Can you work these out from the model? Positions are in its coordinate system, mm. Face numbers are marked on the shaded views. A direction names the side the tool comes from. Coordinates: 2 decimals unless noted, no trailing zeros. Order: outer loops, then holes, each group sorted by start corner. A loop starts at its lowest first (then second) coordinate and runs counter-clockwise, first axis right, second up. Notation, with made-up numbers: (-5, 54.5) -> (13, 54.5) arc R28 ccw to (13, 79.5) -> close; hole circle Ø10 at (46.5, -27.75). An arc over 180 degrees is marked (long way). Return JSON: item names as keys, results as strings. Group by question number.
1) If we section it at A-A, the plane z = -2.5: Please give me the cut outline in (x, y), then the cut area to 3 significant figures.
2) For the marked faces 1 and 2, which set-ups out of +Z, -Z, +X, -X, +Y, -Y let a thin tool reach every point of the face, with its end or its side?
3) For pin 1 (5 mm diameter, centred on x = -14, z = -14, fed in from +Y); pin 2 (4 mm diameter, centred on y = 15.5, z = -8, fed in from -X); pin 3 (10 mm diameter, centred on y = -16, z = -16, fed in from -X); pin 4 (12 mm diameter, centred on x = -0.5, y = 21, fed in from -Z), each with a flat end and sliding along its axis, tell me the tip position at first contact or that it passes through.
4) If I drill on probe 1 along Z at (x, y) = (5.5, -5); probe 2 along Z at (x, y) = (24.5, -13); probe 3 along Y at (x, z) = (25, -3), over which ranges is the centre line in solid material (lowest first)? Write a range as from..to.
5) Thinking about a two-plate mould opening in Y: for the marked faces 3, 4 and 5, which applies, +Y half, -Y half, draft (parallel to the pull), parting line (faces both ways), or undercut?
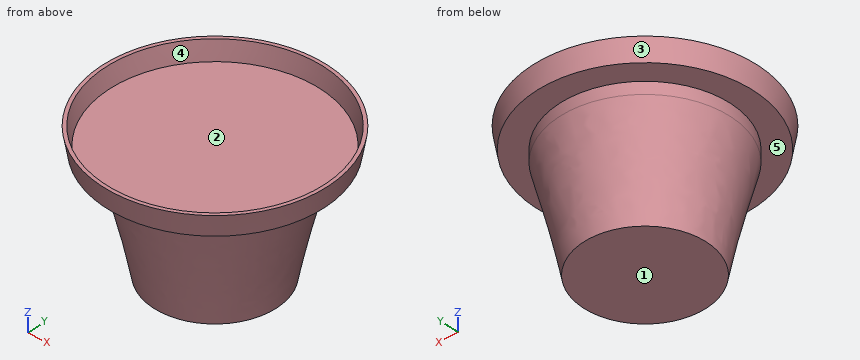
from build123d import *

# Parameters (mm, degrees)
IZIM3_R                     = 25.05
Y_KSEKLIK_EKSTR_ZYON1_DEPTH = 3.5


with BuildPart() as part:
    # Çizim2 → Döndür1 (revolve)
    with BuildSketch(Plane(origin=(0, 0, 0), x_dir=(1, 0, 0), z_dir=(0, 1, 0)), mode=Mode.PRIVATE) as d_nd_r1_sk:
        Polygon((-33, 0), (-31.889140022, 6.3), (-30.889140022, 6.3), (0, 6.3), (0, 5.3), (-30.889140022, 5.3), (-32, 0), align=None)
    revolve(d_nd_r1_sk.sketch.rotate(Axis((0, 0, 0), (0, 0, -1)), 180), axis=Axis((0, 0, 0), (0, 0, -1)))

    # Çizim3 → Yükseklik-Ekstrüzyon1 (add)
    with BuildSketch(Plane(origin=(0, 0, -6.3), x_dir=(-1, 0, 0), z_dir=(0, 0, -1))):
        Circle(IZIM3_R)
    extrude(amount=Y_KSEKLIK_EKSTR_ZYON1_DEPTH)

    # Loft1: read off the stored shape, not the designer's step
    # Loft1: loft between two sections, ruled curve by curve
    loft1_from = [
        Edge.make_bspline([(11.664244151, 13.709318305, -39.8), (-15.754392459, 37.037806607, -39.8), (-39.082880761, 9.619169997, -39.8), (-11.664244151, -13.709318305, -39.8), (15.754392459, -37.037806607, -39.8), (39.082880761, -9.619169997, -39.8), (11.664244151, 13.709318305, -39.8)], [0, 0, 0, 0, 0.5, 0.5, 0.5, 1, 1, 1, 1], 3, [1, 0.333333333, 0.333333333, 1, 0.333333333, 0.333333333, 1]),
    ]
    loft1_to = [
        Edge.make_bspline([(21.774798676, 12.38388641, -9.8), (-2.992974145, 55.933483762, -9.8), (-46.542571497, 31.165710941, -9.8), (-21.774798676, -12.38388641, -9.8), (2.992974145, -55.933483762, -9.8), (46.542571497, -31.165710941, -9.8), (21.774798676, 12.38388641, -9.8)], [0, 0, 0, 0, 0.5, 0.5, 0.5, 1, 1, 1, 1], 3, [1, 0.333333333, 0.333333333, 1, 0.333333333, 0.333333333, 1]),
    ]
    loft1 = Solid(Shell([*[Face.make_surface_from_curves(loft1_from[k], loft1_to[k]) for k in range(1)], Face(Wire(loft1_from)), Face(Wire(loft1_to))]))
    add(loft1)


solid = part.part
Result sheet:
{
 "1": {"outline": "circle Ø65.12 at (0, 0); hole circle Ø62.95 at (0, 0)", "area": "218 mm2"},
 "2": {"face 1": "-Z, +X, -X, +Y, -Y", "face 2": "+Z"},
 "3": {"pin 1": "stops at y = 21.18", "pin 2": "stops at x = -28.43", "pin 3": "stops at x = -21.04", "pin 4": "stops at z = -39.8"},
 "4": {"probe 1": "z = -39.8..-5.3", "probe 2": "z = -6.3..-5.3", "probe 3": "y = -20.72..-18.95, 18.95..20.72"},
 "5": {"face 3": "parting line", "face 4": "undercut", "face 5": "draft"}
}
